Autodesk Fusion 360 part; units mm, degrees
sketch "Sketch1" plane through (0, 0, 0) normal (0, 0, 1) x (1, 0, 0)
  line L0 (0, 0) -> (120, 0)
  line L1 (120, 0) -> (120, 35)
  line L2 (120, 35) -> (0, 35)
  line L3 (0, 35) -> (0, 0)
  dimension "d1" = 120
  dimension "d2" = 35
extrude "Extrude1" add sketch "Sketch1" along normal blind 17.2
chamfer "Chamfer1" distance 7.0437 angle 60 2 edges at (60, 0, 17.2) (60, 35, 17.2) measured on face at (40, 23.3333, 17.2) measured on face at (40, 23.3333, 17.2)
chamfer "Chamfer2" distance 3 angle 45 6 edges at (0, 3.5218, 11.1) (0, 31.4782, 11.1) (0, 17.5, 17.2) (120, 17.5, 17.2) (120, 3.5218, 11.1) (120, 31.4782, 11.1) measured on face at (40, 4.6958, 13.1333) measured on face at (80, 30.3042, 13.1333) measured on face at (40, 20.9854, 17.2) measured on face at (40, 20.9854, 17.2) measured on face at (40, 4.6958, 13.1333) measured on face at (80, 30.3042, 13.1333)
sketch "Sketch2" plane through (0, 0, 0) normal (0, 0, -1) x (1, 0, 0)
  line L0 (0, -0.5773) -> (0, -34.4227)
  line L1 (120, -34.4227) -> (120, -0.5773)
  line L2 (115.1, -7.4) -> (4.9, -7.4)
  line L3 (4.9, -7.4) -> (4.9, -27.6)
  line L4 (4.9, -27.6) -> (115.1, -27.6)
  line L5 (115.1, -27.6) -> (115.1, -7.4)
  line L6 (115.1, -7.4) -> (4.9, -27.6) construction
  line L7 (4.9, -7.4) -> (115.1, -27.6) construction
  line L8 (120, -0.5773) -> (119.5, 0)
  line L9 (0.5, 0) -> (0, -0.5773)
  line L10 (0, -34.4227) -> (0.5, -35)
  line L11 (119.5, -35) -> (120, -34.4227)
  line L12 (60, 0) -> (60, -35) construction
  line L13 (119.5, 0) -> (0.5, 0)
  line L14 (0.5, -35) -> (119.5, -35)
  point P0 (60, -17.5)
  dimension "d9" = 110.2
  dimension "d10" = 20.2
extrude "Extrude2" cut sketch "Sketch2" against normal blind 15.2 contours L2 L3 L4 L5
sketch "Sketch3" plane through (0, 0, 17.2) normal (0, 0, 1) x (-1, 0, 0)
  line L0 (-117, -7.0437) -> (-117, -27.9563)
  line L1 (-117, -27.9563) -> (-3, -27.9563)
  line L2 (-3, -27.9563) -> (-3, -7.0437)
  line L3 (-3, -7.0437) -> (-117, -7.0437)
  line L4 (-60, -27.9563) -> (-60, -7.0437) construction
  line L5 (-117, -17.5) -> (-3, -17.5) construction
  line L6 (-44.8, -11.55) -> (-75.2, -11.55)
  line L7 (-75.2, -11.55) -> (-75.2, -23.45)
  line L8 (-75.2, -23.45) -> (-44.8, -23.45)
  line L9 (-44.8, -23.45) -> (-44.8, -11.55)
  line L10 (-75.2, -11.55) -> (-77.95, -11.55)
  line L11 (-77.95, -11.55) -> (-77.95, -19.45)
  line L12 (-77.95, -19.45) -> (-75.2, -19.45)
  line L13 (-75.2, -19.45) -> (-75.2, -11.55)
  line L14 (-60, -23.45) -> (-60, -11.55) construction
  dimension "d13" = 30.4
  dimension "d14" = 11.9
  dimension "d15" = 2.75
  dimension "d16" = 7.9
extrude "Extrude3" cut sketch "Sketch3" against normal blind 2 contours L6 L7 L8 L9 L13 | L7 L10 L11 L12 L13
equation "d3 = 10 mm - 2.8 mm + 5 mm + 5 mm"
equation "d11 = -5.2 mm - 5 mm - 5 mm"
equation "d13 = 30 mm + 0.4 mm"
equation "d14 = 11.5 mm + 0.4 mm"
equation "d16 = 7.5 mm + 0.4 mm"
Work out the finished part from the listing and answer in its coordinate system (mm). A direction names the side the tool comes from. Give positions to 0.01 mm unless a question says otherwise; leave off trailing zeros. Write each loop counter-clockwise with the first axis right and the second up, starting at its lowest first coordinate (ties: lowest second). Pieces come first, ordered by that corner, then holes. Notation, with made-up numbers: (-32, -11) - (-14, -11) arc R25 ccw to (-14, 6) - close; hole circle Ø5 at (45, 76.25). An arc over 180 degrees is marked (long way). Use one line per item in the form item = value.
1. A cutting plane is placed at C-C (z = 3.25). Write down the section's boundary in (x, y).
Filled in:
outline = (0, 2.45) - (2.13, 0) - (117.87, 0) - (120, 2.45) - (120, 32.55) - (117.87, 35) - (2.13, 35) - (0, 32.55) - close; hole (4.9, 7.4) - (115.1, 7.4) - (115.1, 27.6) - (4.9, 27.6) - close
2. For faces 1 (the face through (44.8, 18, 16)), 2 (the face through (1.48, 31.18, 8.58)), 3 (the face through (115.1, 18, 7)), determine the directions among +Z, -Z, +X, -X, +Y, -Y from which every point of the face is accessible in a straight line to the end or side of a thin tool.
Filled in:
face_1 = +Z, -Z
face_2 = +Z, -X, +Y
face_3 = -Z
3. Consider L1, parallel to X at y = 8.5, z = 6; L2, parallel to Y at x = 64, z = 5; L3, parallel to Z at x = 26.5, y = 8. Determine where each line is inside the solid, lowest interval first.
Filled in:
L1 = 0 to 4.9, 115.1 to 120
L2 = 0 to 7.4, 27.6 to 35
L3 = 15.2 to 17.2
4. Each of these flat-tipped pins is pushed along its axis until it touches: pin 1 Ø16 at (x, y) = (80, 16) entering from -Z; pin 2 Ø4.5 at (x, z) = (76.5, 10) entering from +Y; pin 3 Ø3 at (x, y) = (106.5, 31.5) entering from +Z. Where does it stop, or does it pass through?
Filled in:
pin_1 = 15.2
pin_2 = 33.41
pin_3 = 13.66
5. Determine the mould class of faces 4 (the face through (120, 17, 7)), 5 (the face through (0, 18, 7)), 6 (the face through (59, 29, 0)), 7 (the face through (75.2, 21, 16)) for opening direction X: released by +X, released by -X, zero draft, split by the parting line, or undercut.
Filled in:
face_4 = released by +X
face_5 = released by -X
face_6 = zero draft
face_7 = undercut
6. A cutting plane is placed at B-B (x = 59). Write down the section's boundary in (y, z).
Filled in:
outline = (0, 0) - (7.4, 0) - (7.4, 15.2) - (11.55, 15.2) - (11.55, 17.2) - (7.04, 17.2) - (0, 5) - close; (23.45, 15.2) - (27.6, 15.2) - (27.6, 0) - (35, 0) - (35, 5) - (27.96, 17.2) - (23.45, 17.2) - close
7. A cutting plane is placed at A-A (y = 22). Write down the section's boundary in (x, z), and give its area (3 significant figures).
Filled in:
outline = (0, 0) - (4.9, 0) - (4.9, 15.2) - (44.8, 15.2) - (44.8, 17.2) - (3, 17.2) - (0, 14.2) - close; (75.2, 15.2) - (115.1, 15.2) - (115.1, 0) - (120, 0) - (120, 14.2) - (117, 17.2) - (75.2, 17.2) - close
area = 319 mm^2
8. A cutting plane is placed at D-D (x = 35.5). Write down the section's boundary in (y, z).
Filled in:
outline = (0, 0) - (7.4, 0) - (7.4, 15.2) - (27.6, 15.2) - (27.6, 0) - (35, 0) - (35, 5) - (27.96, 17.2) - (7.04, 17.2) - (0, 5) - close
